The listing builds one solid part. Answer for the finished solid, in the listing's coordinates (mm). A direction names the side the tool comes from. Round coordinates to 2 decimals unless told otherwise and drop trailing zeros. Write each loop counter-clockwise with the first axis right and the second up, starting at its lowest first coordinate (ties: lowest second). Pieces come first, ordered by that corner, then holes. Notation, with made-up numbers: (-8, 41.25) - (23, 41.25) arc R19 ccw to (23, 72.25) - close; hole circle Ø2 at (71.25, -7.75). An arc over 180 degrees is marked (long way). Answer as CSV lines item,"result". Start each with the question number.
Item 1: For a pull along Z with two mould halves and no side action, classify faces 1 (the flat face through (0, -340, -4.762)), 2 (the flat face through (0, -182, 6.35)), 3 (the flat face through (0, -368.3, 5)) as pulls with the +Z half, pulls with the -Z half, needs draft (parallel to the pull), parting line crosses it, or undercut.
Item 2: A cutting plane is placed at A-A on x = 0.5. Determine the outline of the cut face in (y, z).
Item 3: Which of the six approach directions +Z, -Z, +X, -X, +Y, -Y give full straight-line access (tool end or side, diameter ignored) to faces 4 (the flat face through (0, -154, -4.762)), 5 (the flat face through (-6.35, -182, 0))?
Item 4: Straight lines are drawn through the part: line 1 along X through (y, z) = (-331.5, -2); line 2 along Z through (x, y) = (-5.7, -6.35); line 3 along Y through (x, z) = (2.25, -6). For each, find the intervals that lie inside material, in ascending order. Write a range as [from, to].
Item 5: Flat-ended cylindrical pins translate along their axes: pin 1 (0.8 mm diameter, centred on x = 5.5, y = -8.5, fed in from -Z); pin 2 (1.3 mm diameter, centred on x = 0, z = -5.5, fed in from +Y); pin 3 (0.8 mm diameter, centred on x = 2.5, z = -5.5, fed in from -Y). Find the tip coordinate at first contact, or state that the pin passes through.
Item 6: A cutting plane is placed at B-B on y = -290.5. Determine the outline of the cut face in (x, z).
```python
from build123d import *

# Parameters (mm, degrees)
F1_DEPTH = 368.3
F2_R     = 1.190625
F3_DEPTH = 12.701
F4_W     = 12.7
F4_H     = 25.4
F4_H_2   = 12.7
F5_DEPTH = 1.5875


with BuildPart() as f1:
    # F0 (on Front) → F1 (new body)
    with BuildSketch(Plane.XZ):
        Polygon((0, 4.7625), (4.7625, 4.7625), (4.7625, 0), (6.35, 0), (6.35, 6.35), (0, 6.35), align=None)
        Polygon((-4.7625, 4.7625), (0, 4.7625), (0, 6.35), (-6.35, 6.35), (-6.35, -6.35), (6.35, -6.35), (6.35, 0), (4.7625, 0), (4.7625, -4.7625), (-4.7625, -4.7625), align=None)
    extrude(amount=F1_DEPTH)

    # F2 (on face) → F3 (cut, through all)
    with BuildSketch(Plane.YZ.offset(6.35)):
        with Locations((-317.5, 0)):
            Circle(F2_R)
        with Locations((-304.8, 0)):
            Circle(F2_R)
        with Locations((-361.95, 0)):
            Circle(F2_R)
        with Locations((-355.6, 0)):
            Circle(F2_R)
        with Locations((-6.35, 0)):
            Circle(F2_R)
        with Locations((-12.7, 0)):
            Circle(F2_R)
    extrude(amount=-F3_DEPTH, mode=Mode.SUBTRACT)

    # F4 (on face) → F5 (cut, through all)
    with BuildSketch(Plane(origin=(0, 0, -6.35), x_dir=(1, 0, 0), z_dir=(0, 0, -1))):
        with Locations((0, 311.15)):
            Rectangle(F4_W, F4_H)
        with Locations((0, 361.95)):
            Rectangle(F4_W, F4_H_2)
        with Locations((0, 6.35)):
            Rectangle(F4_W, F4_H_2)
    extrude(amount=-F5_DEPTH, mode=Mode.SUBTRACT)


solid = f1.part
```
Geometry says:
1,face 1,"undercut"
1,face 2,"pulls with the +Z half"
1,face 3,"needs draft"
2,outline,"(-368.3, 4.76) - (0, 4.76) - (0, 6.35) - (-368.3, 6.35) - close; (-355.6, -6.35) - (-323.85, -6.35) - (-323.85, -4.76) - (-355.6, -4.76) - close; (-298.45, -6.35) - (-12.7, -6.35) - (-12.7, -4.76) - (-298.45, -4.76) - close"
3,face 4,"+Y, -Y"
3,face 5,"+Z, -Z, -X, +Y, -Y"
4,line 1,"x = [-6.35, -4.76], [4.76, 6.35]"
4,line 2,"z = [-4.76, -1.19], [1.19, 6.35]"
4,line 3,"y = [-355.6, -323.85], [-298.45, -12.7]"
5,pin 1,"stops at z = -4.76"
5,pin 2,"stops at y = -12.7"
5,pin 3,"stops at y = -355.6"
6,outline,"(-6.35, -6.35) - (6.35, -6.35) - (6.35, 6.35) - (-6.35, 6.35) - close; hole (-4.76, -4.76) - (4.76, -4.76) - (4.76, 4.76) - (-4.76, 4.76) - close"
